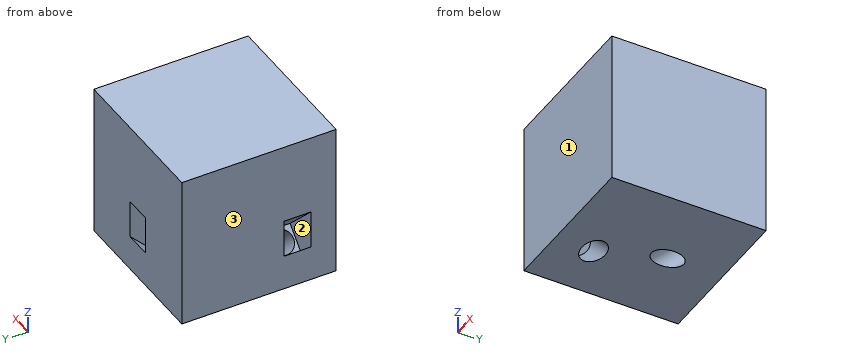
from build123d import *

# Parameters (mm, degrees)
ESQUISSE1_W                  = 40
ESQUISSE1_H                  = 40
BOSS_EXTRU_1_DEPTH           = 40
ESQUISSE2_R                  = 3
ENL_V_MAT_EXTRU_3_DEPTH      = 29.284271247
ENL_V_MAT_EXTRU_3_DEPTH_BACK = 29.284271247
ESQUISSE4_W                  = 7
ESQUISSE4_H                  = 7
ENL_V_MAT_EXTRU_5_DEPTH      = 23.5
ESQUISSE6_R                  = 3
ENL_V_MAT_EXTRU_6_DEPTH      = 29.284271247
ENL_V_MAT_EXTRU_6_DEPTH_BACK = 29.284271247
ESQUISSE7_W                  = 7
ESQUISSE7_H                  = 7
ENL_V_MAT_EXTRU_7_DEPTH      = 23.5


with BuildPart() as part:
    # Esquisse1 → Boss.-Extru.1 (new body)
    with BuildSketch(Plane.XY):
        with Locations((-101.164127838, 15.64516129)):
            Rectangle(ESQUISSE1_W, ESQUISSE1_H)
    extrude(amount=BOSS_EXTRU_1_DEPTH)

    # Esquisse2 → Enlèv. mat.-Extru.3 (cut, two sides)
    with BuildSketch(Plane(origin=(0, 17.822580645, 17.822580645), x_dir=(1, 0, 0), z_dir=(0, 0.707106781, 0.707106781))) as enl_v_mat_extru_3_sk:
        with Locations((-101.164127838, 15.204935265)):
            Circle(ESQUISSE2_R)
    extrude(amount=ENL_V_MAT_EXTRU_3_DEPTH, mode=Mode.SUBTRACT)
    extrude(enl_v_mat_extru_3_sk.sketch, amount=-ENL_V_MAT_EXTRU_3_DEPTH_BACK, mode=Mode.SUBTRACT)

    # Esquisse4 → Enlèv. mat.-Extru.5 (cut)
    with BuildSketch(Plane(origin=(0, 17.822580645, 17.822580645), x_dir=(1, 0, 0), z_dir=(0, 0.707106781, 0.707106781))):
        with Locations((-101.164127838, 15.204935265)):
            Rectangle(ESQUISSE4_W, ESQUISSE4_H)
    extrude(amount=ENL_V_MAT_EXTRU_5_DEPTH, mode=Mode.SUBTRACT)

    # Esquisse6 → Enlèv. mat.-Extru.6 (cut, two sides)
    with BuildSketch(Plane(origin=(-60.582063919, 0, 60.582063919), x_dir=(-0.707106781, 0, -0.707106781), z_dir=(0.707106781, 0, -0.707106781))) as enl_v_mat_extru_6_sk:
        with Locations((75.67597643, 5.64516129)):
            Circle(ESQUISSE6_R)
    extrude(amount=ENL_V_MAT_EXTRU_6_DEPTH, mode=Mode.SUBTRACT)
    extrude(enl_v_mat_extru_6_sk.sketch, amount=-ENL_V_MAT_EXTRU_6_DEPTH_BACK, mode=Mode.SUBTRACT)

    # Esquisse7 → Enlèv. mat.-Extru.7 (cut)
    with BuildSketch(Plane(origin=(-60.582063919, 0, 60.582063919), x_dir=(-0.707106781, 0, -0.707106781), z_dir=(0.707106781, 0, -0.707106781))):
        with Locations((75.67597643, 5.64516129)):
            Rectangle(ESQUISSE7_W, ESQUISSE7_H)
    extrude(amount=-ENL_V_MAT_EXTRU_7_DEPTH, mode=Mode.SUBTRACT)


solid = part.part
Can you work these out from the model? Positions are in its coordinate system, mm. Face numbers are marked on the shaded views. Coordinates: 2 decimals unless noted, no trailing zeros. Write each loop counter-clockwise with the first axis right and the second up, starting at its lowest first coordinate (ties: lowest second). Pieces come first, ordered by that corner, then holes. Notation, with made-up numbers: M 20,85.25 L 27,85.25 A24 cw 27,113.25 Z; hole C 85,66 d2. An arc over 180 degrees is marked long. Use one line per item in the form item = value.
Q1. I need wall thicknesses on line 1 along X through (y, z) = (8.5, 11); line 2 along Z through (x, y) = (-107, 4.5); line 3 along X through (y, z) = (9, 9.5). Which ranges of each line are inside material? Lowest first, please. Write a range as from..to.
Model answer:
line_1 = -113.07..-81.16
line_2 = 3.9..40
line_3 = -111.66..-81.16
Q2. If we section it at D-D (z = 4): State how many separate pieces and enclosed holes the cut face has, then the cut area to 3 significant figures.
Model answer:
separate_pieces = 1
enclosed_holes = 2
area = 1,520 mm^2
Q3. If we section it at C-C (z = 12): Write out the boundary of the cut face in (x, y).
Model answer:
outline = M -121.16,-4.35 L -81.16,-4.35 L -81.16,35.65 L -97.66,35.65 L -97.66,28.55 L -104.66,28.55 L -104.66,35.65 L -121.16,35.65 L -121.16,9.15 L -114.07,9.15 L -114.07,2.15 L -121.16,2.15 Z
Q4. If we section it at A-A (x = -102): Write out the boundary of the cut face in (y, z), then the cut area to 3 significant figures.
Model answer:
outline = M -4.35,0 L 17.43,0 L 26.54,9.11 L 26.1,9.55 L 35.65,19.09 L 35.65,40 L -4.35,40 Z; M 25.58,0 L 35.65,0 L 35.65,9.19 L 31.05,4.6 L 30.61,5.03 Z
area = 1,470 mm^2
Q5. If we section it at B-B (y = 8): Write out the boundary of the cut face in (x, z), then the cut area to 3 significant figures.
Model answer:
outline = M -121.16,0 L -109.65,0 L -115.41,5.76 L -116.57,4.6 L -121.16,9.19 Z; M -121.16,19.09 L -111.62,9.55 L -112.78,8.39 L -104.39,0 L -81.16,0 L -81.16,40 L -121.16,40 Z
area = 1,490 mm^2
Q6. We'd pull the mould along Y, two halves only. Please class the marked faces 1, 2 and 3: +Y half, -Y half, draft (parallel to the pull), parting line (faces both ways), or undercut.
Model answer:
face_1 = -Y half
face_2 = undercut
face_3 = draft
